Study the drawing (mm; zero at the part's minimum x, y, z) and answer. A direction names the side the tool comes from. Coordinates: 2 decimals unless noted, no trailing zeros. Loops run counter-clockwise (first coordinate to the right, second up) from the corner with the lowest first, then second, coordinate; pieces in that order, holes last. Notation, with made-up numbers: (-33, 34.5) - (15, 34.5) arc R21 cw to (15, 39.5) - close; hole circle Ø2 at (-26, 70). An arc over 180 degrees is marked (long way). Put each result on its own line as item: value.
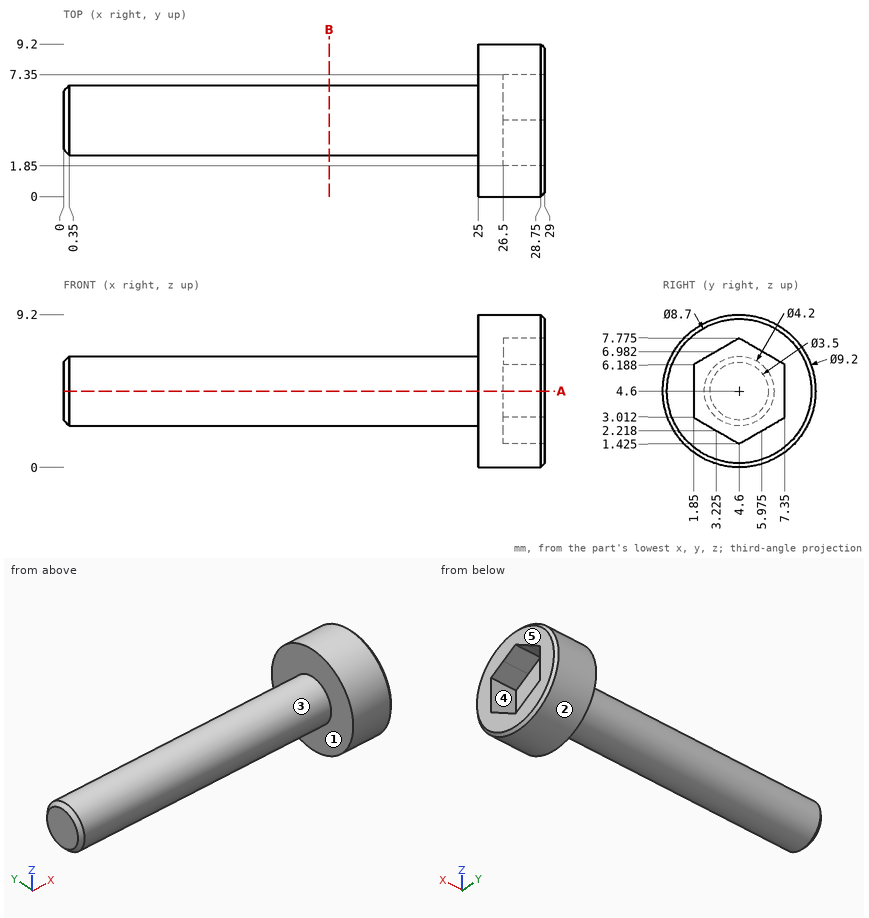
1) For the marked faces 1 and 2, determine the directions among +Z, -Z, +X, -X, +Y, -Y from which every point of the face is accessible in a straight line to the end or side of a thin tool.
Found:
face 1: -X
face 2: +X, -X
2) The part is cut by section A-A (z = 4.6). Give the vertices of the cut face in (x, y), and give its area (3 significant figures).
Found:
outline: (0, 2.85) - (0.35, 2.5) - (25, 2.5) - (25, 0) - (28.75, 0) - (29, 0.25) - (29, 1.85) - (26.5, 1.85) - (26.5, 7.35) - (29, 7.35) - (29, 8.95) - (28.75, 9.2) - (25, 9.2) - (25, 6.7) - (0.35, 6.7) - (0, 6.35) - close
area: 128 mm^2
3) The part is cut by section B-B (x = 16). Give the vertices of the cut face in (y, z).
Found:
outline: circle Ø4.2 at (4.6, 4.6)
4) Each of these flat-tipped pins is pushed along its axis until it touches: pin 1 (3 mm diameter, centred on y = 6, z = 6.5, fed in from -X); pin 2 (3 mm diameter, centred on y = 5.5, z = 5, fed in from +X); pin 3 (1 mm diameter, centred on x = 24, y = 7, fed in from -Z) (1 decimal); pin 4 (5 mm diameter, centred on x = 15, z = 1, fed in from +Y). Where does it stop, or does it pass through?
Found:
pin 1: stops at x = 0
pin 2: stops at x = 26.5
pin 3: stops at z = 3.7
pin 4: stops at y = 6.39
5) Straight lines are drawn through the part: L1, parallel to X at y = 1, z = 2.75; L2, parallel to X at y = 3.5, z = 2.5; L3, parallel to Z at x = 17.5, y = 5. For each, find the intervals that lie inside material, in ascending order. Write a range as [from, to].
Found:
L1: x = [25, 29]
L2: x = [25, 26.5]
L3: z = [2.54, 6.66]
6) For a pull along Z with two mould halves and no side action, classify the marked faces 3, 4 and 5 as pulls with the +Z half, pulls with the -Z half, needs draft (parallel to the pull), parting line crosses it, or undercut.
Found:
face 3: parting line crosses it
face 4: undercut
face 5: needs draft
